Source: three-view drawing plus pictorial views. Frame: mm from the lowest corner of the part. Give positions to 0.01 mm unless a question says otherwise; leave off trailing zeros. Write each loop counter-clockwise with the first axis right and the second up, starting at its lowest first coordinate (ties: lowest second). Pieces come first, ordered by that corner, then holes.
Q1. Cut plane B-B on y = 24.9. Return the cut outline in (x, z).
Q2. Cut plane A-A on x = 24.9. Return the cut outline in (y, z).
Q3. Cut plane C-C on z = 1. Count the separate pieces of the cut face and the enclosed holes in it, plus the area to 3 significant figures.
Q4. Line query: L1, parallel to X at y = 16, z = 0.25; L2, parallel to Y at x = 20.5, z = 0.35; L3, parallel to Y at x = 30, z = 0.95. Output: solid intervals per line, ascending.
Q5. Pin query (flat end, axial travel): pin 1 (5.5 mm diameter, centred on x = 34.6, y = 14.9, fed in from +Z); pin 2 (0.7 mm diameter, centred on y = 49, z = 2, fed in from -X); pin 3 (1.2 mm diameter, centred on y = 2, z = 1, fed in from +X); pin 4 (0.7 mm diameter, centred on x = 2, z = 1.5, fed in from +Y). Return the tip coordinate at first contact, or that it passes through.
Q6. Cut plane D-D on x = 11.1. Return the cut outline in (y, z).
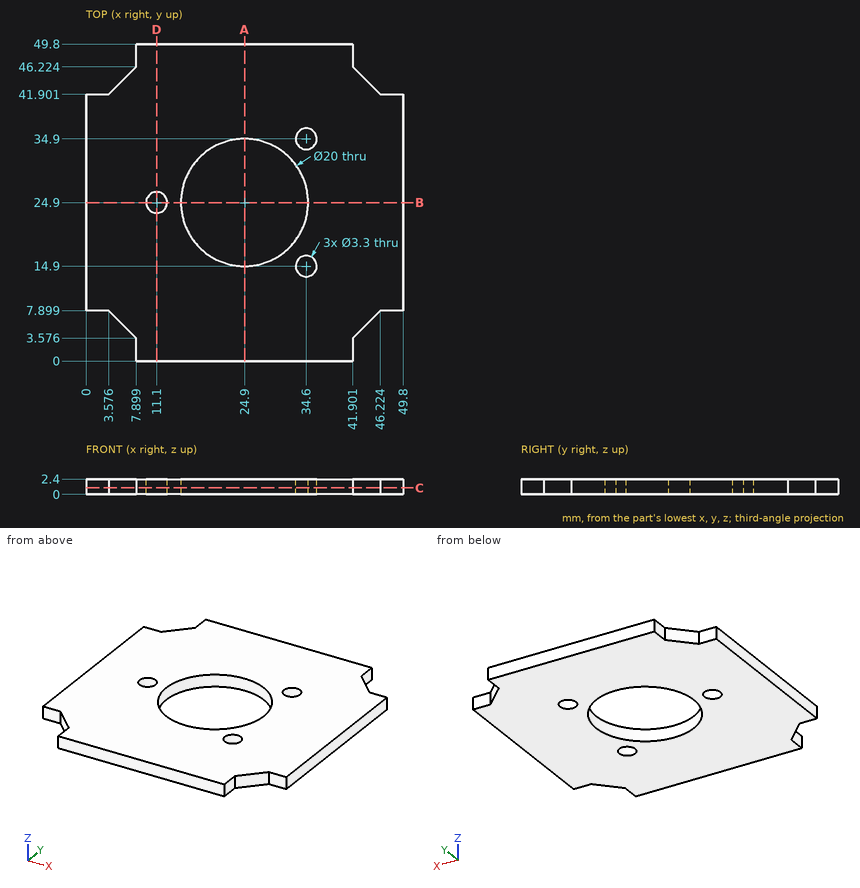
Data:
1. outline: (0, 0) - (9.45, 0) - (9.45, 2.4) - (0, 2.4) - close; (12.75, 0) - (14.9, 0) - (14.9, 2.4) - (12.75, 2.4) - close; (34.9, 0) - (49.8, 0) - (49.8, 2.4) - (34.9, 2.4) - close
2. outline: (0, 0) - (14.9, 0) - (14.9, 2.4) - (0, 2.4) - close; (34.9, 0) - (49.8, 0) - (49.8, 2.4) - (34.9, 2.4) - close
3. separate pieces: 1
3. enclosed holes: 4
3. area: 1,930 mm2
4. L1: x = 0 to 20.34, 29.46 to 33.37, 35.83 to 49.8
4. L2: y = 0 to 15.92, 33.88 to 49.8
4. L3: y = 0 to 16.3, 33.5 to 49.8
5. pin 1: stops at z = 2.4
5. pin 2: stops at x = 7.9
5. pin 3: stops at x = 41.9
5. pin 4: stops at y = 41.9
6. outline: (0, 0) - (23.25, 0) - (23.25, 2.4) - (0, 2.4) - close; (26.55, 0) - (49.8, 0) - (49.8, 2.4) - (26.55, 2.4) - close
